For this review, use the dimensioned drawing (mm, ordinates from the lowest corner) and the shaded views. A direction names the side the tool comes from. Coordinates: 2 decimals unless noted, no trailing zeros. Write each loop counter-clockwise with the first axis right and the second up, starting at its lowest first coordinate (ties: lowest second). Pieces come first, ordered by that corner, then holes. Notation, with made-up numbers: (66, 31.25) - (117, 31.25) arc R12 cw to (117, 47.25) - close; hole circle Ø2 at (-33.75, -5.75). An arc over 180 degrees is marked (long way). Put each result on its own line as item: value.
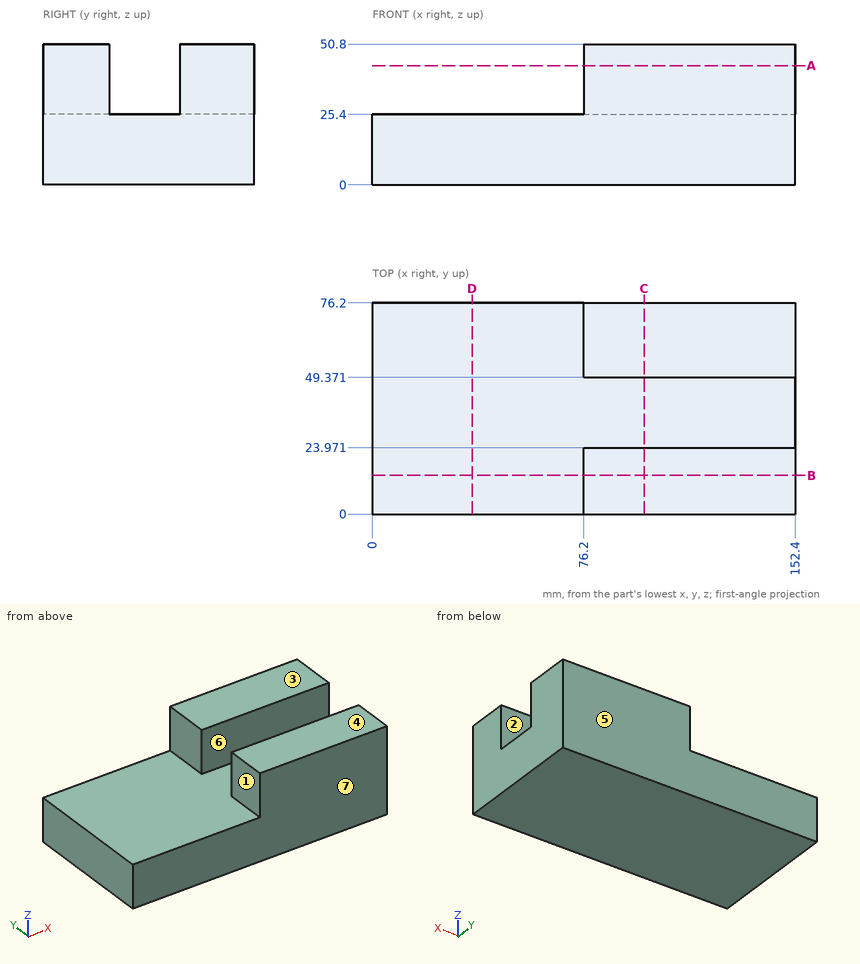
1. Machinability: for the marked faces 1, 2 and 3, which of the approach directions +Z, -Z, +X, -X, +Y, -Y give a long, thin tool a straight path to every point of the face, cutting with its end or side? Answer none if there is none.
Determined:
face 1: +Z, -X, +Y, -Y
face 2: +Z, +X, -X
face 3: +Z, +X, -X, +Y, -Y
2. Consider section C-C on x = 98. State the section outline as (y, z) points.
Determined:
outline: (0, 0) - (76.2, 0) - (76.2, 50.8) - (49.37, 50.8) - (49.37, 25.4) - (23.97, 25.4) - (23.97, 50.8) - (0, 50.8) - close
3. To check wall thickness, follow probe 1 along Y at (x, z) = (143, 26.5); probe 2 along Z at (x, y) = (31.5, 36); probe 3 along X at (y, z) = (50, 33.5). State the ranges of each line that lie inside material, in increasing order.
Determined:
probe 1: y = 0 to 23.97, 49.37 to 76.2
probe 2: z = 0 to 25.4
probe 3: x = 76.2 to 152.4
4. Consider section D-D on x = 36. State the section outline as (y, z) points, plus the area to 3 significant figures.
Determined:
outline: (0, 0) - (76.2, 0) - (76.2, 25.4) - (0, 25.4) - close
area: 1,940 mm^2
5. Consider section B-B on y = 14. State the section outline as (x, z) points, plus the area to 3 significant figures.
Determined:
outline: (0, 0) - (152.4, 0) - (152.4, 50.8) - (76.2, 50.8) - (76.2, 25.4) - (0, 25.4) - close
area: 5,810 mm^2
6. Consider section A-A on z = 43. State the section outline as (x, y) points.
Determined:
outline: (76.2, 0) - (152.4, 0) - (152.4, 23.97) - (76.2, 23.97) - close; (76.2, 49.37) - (152.4, 49.37) - (152.4, 76.2) - (76.2, 76.2) - close
7. The part is to be moulded in two halves that separate along Y. For the marked faces 4, 5, 6 and 7, say which applies: +Y half, -Y half, draft (parallel to the pull), parting line (faces both ways), or undercut.
Determined:
face 4: draft
face 5: +Y half
face 6: undercut
face 7: -Y half
8. For pin 1 Ø12 at (y, z) = (7.5, 41.5) entering from -X, flat-tipped, find the tip position at first contact; note if it passes through.
Determined:
pin 1: stops at x = 76.2
